Could you check a few things on this model? Use its own coordinates, in mm. Coordinates: 2 decimals unless noted, no trailing zeros. Order: outer loops, then holes, each group sorted by start corner. A loop starts at its lowest first (then second) coordinate and runs counter-clockwise, first axis right, second up. Notation, with made-up numbers: (-7, 67.25) - (24, 67.25) arc R11 cw to (24, 82.25) - close; hole circle Ø7 at (-30, -18.75). An arc over 180 degrees is marked (long way). Answer as a JSON object with one key per item and string values. Group by question number.
(1) Imagine slicing it at A-A, the plane y = 0. Write out the boundary of the cut face in (x, z) (3 decimals), and give its area (3 significant figures).
(2) Please list where these lines run through material, in increasing order: probe 1 along Y at (x, z) = (0, -38); probe 2 along Z at (x, y) = (-10.5, 29); probe 3 along Y at (x, z) = (-13, -3.5).
(3) Imagine slicing it at C-C, the plane z = -34.5. Write out the boundary of the cut face in (x, y), and give its area (3 significant figures).
(4) Imagine slicing it at D-D, the plane z = 8. Write out the boundary of the cut face in (x, y) (3 decimals).
(5) We'd pull the mould along X, two halves only. Please class faces 1 (the cylindrical face through (16.72, 5.26, -40.5)), 2 (the flat face through (9, 29, 0)), 3 (the cylindrical face through (-3.902, 29.717, -47.584)): pulls with the +X half, pulls with the -X half, needs draft (parallel to the pull), parting line crosses it, or undercut.
(6) Will these pins go through, and if not, where does the flat tip stop? P1, Ø1.5, axis at x = 8.5, y = -18, coming from the -Z side; P2, Ø5, axis at x = 4.5, y = 18.5, coming from the -Z side; P3, Ø10, axis at x = 30.5, y = 6, coming from the -Z side.
from build123d import *

# Parameters (mm, degrees)
F0_R     = 29.972
F1_DEPTH = 101.6
F2_R     = 47.625
F3_DEPTH = 19.05
F4_R     = 17.526
F5_DEPTH = 120.651
F6_SIZE  = 5.08
F7_R     = 5.08


with BuildPart() as f1:
    # F0 (on Top) → F1 (new body)
    with BuildSketch(Plane.XY):
        Circle(F0_R)
    extrude(amount=-F1_DEPTH)

    # F2 (on Top) → F3 (join)
    with BuildSketch(Plane.XY):
        Circle(F2_R)
    extrude(amount=F3_DEPTH)

    # F4 (on face) → F5 (cut, through all)
    with BuildSketch(Plane.XY.offset(19.05)):
        Circle(F4_R)
    extrude(amount=-F5_DEPTH, mode=Mode.SUBTRACT)

    # F6
    f6_edges = [f1.edges().sort_by_distance(p)[0] for p in [
        (-29.972, 0, -101.6),
        (-47.625, 0, 0),
        (-47.625, 0, 19.05),
    ]]
    chamfer(f6_edges, length=F6_SIZE)

    # F7
    f7_edges = [f1.edges().sort_by_distance(p)[0] for p in [
        (-17.526, 0, 19.05),
        (-17.526, 0, -101.6),
    ]]
    fillet(f7_edges, radius=F7_R)


solid = f1.part
Result set:
{
 "1": {"outline": "(-47.625, 5.08) - (-42.545, 0) - (-29.972, 0) - (-29.972, -96.52) - (-24.892, -101.6) - (-22.606, -101.6) arc R5.08 ccw to (-17.526, -96.52) - (-17.526, 13.97) arc R5.08 ccw to (-22.606, 19.05) - (-42.545, 19.05) - (-47.625, 13.97) - close; (17.526, -96.52) arc R5.08 ccw to (22.606, -101.6) - (24.892, -101.6) - (29.972, -96.52) - (29.972, 0) - (42.545, 0) - (47.625, 5.08) - (47.625, 13.97) - (42.545, 19.05) - (22.606, 19.05) arc R5.08 ccw to (17.526, 13.97) - close", "area": "3,580 mm^2"},
 "2": {"probe 1": "y = -29.97 to -17.53, 17.53 to 29.97", "probe 2": "z = 0 to 19.05", "probe 3": "y = -27.01 to -11.75, 11.75 to 27.01"},
 "3": {"outline": "circle Ø59.94 at (0, 0); hole circle Ø35.05 at (0, 0)", "area": "1,860 mm^2"},
 "4": {"outline": "circle Ø95.25 at (0, 0); hole circle Ø35.052 at (0, 0)"},
 "5": {"face 1": "undercut", "face 2": "needs draft", "face 3": "parting line crosses it"},
 "6": {"P1": "stops at z = -101.21", "P2": "stops at z = -101.49", "P3": "stops at z = -100.41"}
}
